CAD build for the part. Positions are in the model's coordinates, mm. A direction names the side the tool comes from. Give positions to 0.01 mm unless a question says otherwise; leave off trailing zeros. Order: outer loops, then holes, each group sorted by start corner. A loop starts at its lowest first (then second) coordinate and runs counter-clockwise, first axis right, second up.
from build123d import *

# Parameters (mm, degrees)
F_3_16_0_1875_DIAMETER_HOLE1_D = 4.7625
FILLET1_R                      = 2.54
CHAMFER1_SIZE                  = 1.27


with BuildPart() as part:
    # Sketch1 → Revolve1 (revolve)
    with BuildSketch(Plane(origin=(0, 0, 0), x_dir=(0, 0, -1), z_dir=(1, 0, 0))):
        Polygon((0, 22.863953603), (19.05, 9.525), (19.05, 31.75), (5.08, 31.75), (5.08, 44.45), (0, 44.45), align=None)
    revolve(axis=Axis((0, 0, 18.454150881), (0, 0, -1)))

    # 3/16 (0.1875) Diameter Hole1 (through all)
    with Locations(Plane.XY):
        with Locations((0, 38.1), (38.1, 0), (0, -38.1), (-38.1, 0), (0, 0)):
            Hole(F_3_16_0_1875_DIAMETER_HOLE1_D / 2)

    # Fillet1
    fillet1_edges = [part.edges().sort_by_distance(p)[0] for p in [
        (0, -31.75, -5.08),
    ]]
    fillet(fillet1_edges, radius=FILLET1_R)

    # Chamfer1
    chamfer1_edges = [part.edges().sort_by_distance(p)[0] for p in [
        (0, -31.75, -19.05),
        (0, -44.45, -5.08),
    ]]
    chamfer(chamfer1_edges, length=CHAMFER1_SIZE)


solid = part.part
1. Mould opens along X. For faces 1 (the cylindrical face through (0.31, -35.74, -2.58)), 2 (the flat face through (-19, 19, 0)), 3 (the cylindrical face through (13.352, 42.397, -1.878)) say: released by +X, released by -X, zero draft, split by the parting line, or undercut.
2. Saw through at C-C on z = -13. Give the cut face in (x, y).
3. Saw through at A-A on x = 0. Give the cut face in (y, z) (3 decimals).
4. Wall check: line 1 (X direction, y = -1, z = -5); line 2 (Z direction, x = 12.5, y = 32); line 3 (Y direction, x = -3, z = -16.75). Give the ranges that are in metal, low to high.
5. Pin check, flat tips, straight feed: P1, Ø5.5, axis at x = 0, y = -38.1, coming from the -Z side; P2, Ø8, axis at y = -28, z = -11, coming from the +X side; P3, Ø3, axis at y = 24, z = -12, coming from the -X side; P4, Ø3, axis at x = 0, y = 38.1, coming from the +Z side. Stop position of each tip, or through.
6. 3-axis set-ups, long thin cutter, end or side, ignore diameter. For faces 4 (the cylindrical face through (40.48, 0.1, -2.58)), 5 (the flat face through (-29, -19, -5.08)): which of +Z, -Z, +X, -X, +Y, -Y reach the whole face in a straight line?
Reported:
1. face 1: undercut
1. face 2: zero draft
1. face 3: split by the parting line
2. outline: circle Ø63.5 at (0, 0); hole circle Ø27.52 at (0, 0)
3. outline: (-44.45, -3.81) - (-43.18, -5.08) - (-40.481, -5.08) - (-40.481, 0) - (-44.45, 0) - close; (-35.719, -5.08) - (-34.29, -5.08) arc R2.54 cw to (-31.75, -7.62) - (-31.75, -17.78) - (-30.48, -19.05) - (-9.525, -19.05) - (-22.864, 0) - (-35.719, 0) - close; (9.525, -19.05) - (30.48, -19.05) - (31.75, -17.78) - (31.75, -7.62) arc R2.54 cw to (34.29, -5.08) - (35.719, -5.08) - (35.719, 0) - (22.864, 0) - close; (40.481, -5.08) - (43.18, -5.08) - (44.45, -3.81) - (44.45, 0) - (40.481, 0) - close
4. line 1: x = -43.25 to -40.26, -35.94 to -19.34, 19.34 to 35.94, 40.26 to 43.25
4. line 2: z = -5.08 to 0
4. line 3: y = -31.61 to -10.72, 10.72 to 31.61
5. P1: stops at z = -5.08
5. P2: stops at x = 20.79
5. P3: stops at x = -22.4
5. P4: passes through
6. face 4: +Z, -Z
6. face 5: -Z
